Verification items for the finished model (mm, model axes). Coordinates: 2 decimals unless noted, no trailing zeros. Order: outer loops, then holes, each group sorted by start corner. A loop starts at its lowest first (then second) coordinate and runs counter-clockwise, first axis right, second up. Notation, with made-up numbers: M -40,25.25 L -25,25.25 A17 cw -25,34.25 Z; hole C -27,7 d9. An arc over 180 degrees is marked long. Return JSON: item names as keys, results as strings. Group by question number.
Q1. Thickness scan on probe 1 along Y at (x, z) = (23.6, 0); probe 2 along Y at (x, z) = (24.6, 0); probe 3 along Y at (x, z) = (2, -9.5). Record the ranges inside material, lowest first.
Q2. Go/stop test with flat-tipped pins: pin 1 Ø2.5 at (y, z) = (25.02, 12.5) entering from +X; pin 2 Ø12 at (y, z) = (20, -1) entering from -X; pin 3 Ø12 at (x, z) = (-16, -7) entering from +Y. Record where each tip stops, or that it passes through.
Q3. Section check A-A, the plane y = 25.02. Enter the section's corners in (x, z).
Q4. Section check C-C, the plane x = 9. Enter the section's corners in (y, z), then the cut area to 3 significant figures.
Q5. Section check B-B, the plane z = 12.5. Enter the section's corners in (x, y), then the cut area to 3 significant figures.
Q6. Mould release check, pull along Y, two halves, no side actions. Record for faces 1 (the face through (23, 26, 5)), 2 (the face through (24.014, 11.056, 0.325)), 3 (the face through (-2, 1, 0)): pulls with the +Y half, pulls with the -Y half, needs draft (parallel to the pull), parting line crosses it, or undercut.
Q7. Section check D-D, the plane z = 6. Enter the section's corners in (x, y), then the cut area to 3 significant figures.
from build123d import *

# Parameters (mm, degrees)
RESSALTO_EXTRUS_O1_DEPTH  = 20
ESBO_O2_R                 = 3
CORTE_EXTRUS_O1_DEPTH     = 50
CONVERTER_S_LIDO1_START   = -21
CONVERTER_S_LIDO1_DEPTH   = 41
CONVERTER_S_LIDO1_START_2 = -20
CONVERTER_S_LIDO1_2_DEPTH = 40
ESBO_O3_R                 = 2
CORTE_EXTRUS_O2_DEPTH     = 10
ESBO_O4_R                 = 1.5
CORTE_EXTRUS_O3_DEPTH     = 8


with BuildPart() as part:
    # Esboço1 → Ressalto-extrusão1 (new, symmetric)
    with BuildSketch(Plane.XY):
        Polygon((23, 49), (23, 1), (-25, 1), (-25, -1), (23, -1), (25, -1), (25, 1), (25, 49), align=None)
    extrude(amount=RESSALTO_EXTRUS_O1_DEPTH, both=True)

    # Esboço2 → Corte-extrusão1 (cut)
    with BuildSketch(Plane(origin=(25, 0, 0), x_dir=(0, 0, -1), z_dir=(1, 0, 0))):
        with Locations((0, 25.02)):
            Circle(ESBO_O2_R)
    extrude(amount=-CORTE_EXTRUS_O1_DEPTH, mode=Mode.SUBTRACT)

    # Converter-Sólido1: read off the stored shape, not the designer's step
    # Converter-Sólido1 outline → Converter-Sólido1 (cut)
    with BuildSketch(Plane.XY.offset(CONVERTER_S_LIDO1_START)):
        with BuildLine():
            Line((25, -1), (25, 3))
            ThreePointArc((25, 3), (23.828427125, 0.171572875), (21, -1))
            Line((21, -1), (25, -1))
        make_face()
    extrude(amount=CONVERTER_S_LIDO1_DEPTH, mode=Mode.SUBTRACT)

    # Converter-S_lido1 2 outline → Converter-S_lido1 2 (add)
    with BuildSketch(Plane.XY.offset(CONVERTER_S_LIDO1_START_2)):
        with BuildLine():
            Line((23, 1), (23, 3))
            ThreePointArc((23, 3), (22.414213562, 1.585786438), (21, 1))
            Line((21, 1), (23, 1))
        make_face()
    extrude(amount=CONVERTER_S_LIDO1_2_DEPTH)

    # Esboço3 → Corte-extrusão2 (cut)
    with BuildSketch(Plane.XZ.offset(1)):
        with Locations(Location((9, 12.5, 0), (0, 0, 270))):
            Circle(ESBO_O3_R)
        with Locations(Location((9, -12.5, 0), (0, 0, 270))):
            Circle(ESBO_O3_R)
        with Locations(Location((-12.650635095, 0, 0), (0, 0, 270))):
            Circle(ESBO_O3_R)
    extrude(amount=-CORTE_EXTRUS_O2_DEPTH, mode=Mode.SUBTRACT)

    # Esboço4 → Corte-extrusão3 (cut)
    with BuildSketch(Plane(origin=(25, 0, 0), x_dir=(0, 0, -1), z_dir=(1, 0, 0))):
        with Locations((0, 37.52)):
            Circle(ESBO_O4_R)
        with Locations((12.5, 25.02)):
            Circle(ESBO_O4_R)
        with Locations((0, 12.52)):
            Circle(ESBO_O4_R)
        with Locations((-12.5, 25.02)):
            Circle(ESBO_O4_R)
    extrude(amount=-CORTE_EXTRUS_O3_DEPTH, mode=Mode.SUBTRACT)


solid = part.part
Numbers:
{
 "1": {"probe 1": "y = -0.04 to 11.02, 14.02 to 22.02, 28.02 to 36.02, 39.02 to 49", "probe 2": "y = 1.26 to 11.02, 14.02 to 22.02, 28.02 to 36.02, 39.02 to 49", "probe 3": "y = -1 to 1"},
 "2": {"pin 1": "passes through", "pin 2": "stops at x = 23", "pin 3": "stops at y = 1"},
 "3": {"outline": "M 23,-20 L 25,-20 L 25,-14 L 23,-14 Z; M 23,-11 L 25,-11 L 25,-3 L 23,-3 Z; M 23,3 L 25,3 L 25,11 L 23,11 Z; M 23,14 L 25,14 L 25,20 L 23,20 Z"},
 "4": {"outline": "M -1,-20 L 1,-20 L 1,-14.5 L -1,-14.5 Z; M -1,-10.5 L 1,-10.5 L 1,10.5 L -1,10.5 Z; M -1,14.5 L 1,14.5 L 1,20 L -1,20 Z", "area": "64.0 mm2"},
 "5": {"outline": "M -25,-1 L 7,-1 L 7,1 L -25,1 Z; M 11,-1 L 21,-1 A4 ccw 25,3 L 25,23.52 L 23,23.52 L 23,3 A2 cw 21,1 L 11,1 Z; M 23,26.52 L 25,26.52 L 25,49 L 23,49 Z", "area": "179 mm2"},
 "6": {"face 1": "needs draft", "face 2": "undercut", "face 3": "pulls with the +Y half"},
 "7": {"outline": "M -25,-1 L 21,-1 A4 ccw 25,3 L 25,49 L 23,49 L 23,3 A2 cw 21,1 L -25,1 Z", "area": "193 mm2"}
}
